from build123d import *

# Parameters (mm, degrees)
SKETCH1_W            = 20
SKETCH1_H            = 14.4
BOSS_EXTRUDE1_DEPTH  = 1.8
SKETCH2_W            = 20
SKETCH2_H            = 10
BOSS_EXTRUDE2_DEPTH  = 2.1
SKETCH3_W            = 30
SKETCH3_H            = 20
BOSS_EXTRUDE3_DEPTH  = 3
SKETCH4_W            = 2
SKETCH4_H            = 15
BOSS_EXTRUDE4_DEPTH  = 0.8
FILLET1_R            = 1.5
SKETCH5_W            = 27
SKETCH5_H            = 3
BOSS_EXTRUDE6_DEPTH  = 10
CUT_EXTRUDE1_DEPTH   = 40.819718733
SKETCH7_W            = 20
SKETCH7_H            = 4
BOSS_EXTRUDE7_DEPTH  = 4
SKETCH8_W            = 20
SKETCH8_H            = 4
BOSS_EXTRUDE8_DEPTH  = 4
FILLET3_R            = 2
FILLET2_R            = 1
FILLET4_R            = 1
SKETCH10_W           = 7
SKETCH10_H           = 4
BOSS_EXTRUDE10_DEPTH = 7
SKETCH11_W           = 3
SKETCH11_H           = 7
BOSS_EXTRUDE11_DEPTH = 3
FILLET5_R            = 2
FILLET6_R            = 1
FILLET7_R            = 3


# Some blends are built 0.0001 mm under size
with BuildPart() as part:
    # Sketch1 → Boss-Extrude1 (new body)
    with BuildSketch(Plane(origin=(0, 0, 0), x_dir=(1, 0, 0), z_dir=(0, 1, 0))):
        with Locations((10, -7.2)):
            Rectangle(SKETCH1_W, SKETCH1_H)
    extrude(amount=BOSS_EXTRUDE1_DEPTH)

    # Sketch2 → Boss-Extrude2 (add)
    with BuildSketch(Plane(origin=(0, 1.8, 0), x_dir=(1, 0, 0), z_dir=(0, 1, 0))):
        with Locations((10, -7.2)):
            Rectangle(SKETCH2_W, SKETCH2_H)
    extrude(amount=BOSS_EXTRUDE2_DEPTH)

    # Sketch3 → Boss-Extrude3 (add)
    with BuildSketch(Plane(origin=(0, 3.9, 0), x_dir=(1, 0, 0), z_dir=(0, 1, 0))):
        with Locations((15, -7.2)):
            Rectangle(SKETCH3_W, SKETCH3_H)
    extrude(amount=BOSS_EXTRUDE3_DEPTH)

    # Sketch4 → Boss-Extrude4 (add)
    with BuildSketch(Plane(origin=(0, 3.9, 0), x_dir=(-1, 0, 0), z_dir=(0, -1, 0))):
        with Locations((-28, -7.2)):
            Rectangle(SKETCH4_W, SKETCH4_H)
    extrude(amount=BOSS_EXTRUDE4_DEPTH)

    # Fillet1
    # the kernel refuses this fillet: 1.5 mm, written as the material it takes off along each edge
    with BuildSketch(Plane(origin=(27, 3.1, -3.61662479), x_dir=(0, 1, 0), z_dir=(0, 0, 1))) as fillet1_piece_1:
        with BuildLine():
            CenterArc((1.5, -1.326649916), FILLET1_R, 117.818139285, 62.181860715)
            Line((0, -1.326649916), (-0.03, -1.326649916))
            Line((-0.03, -1.326649916), (-0.03, 0))
            Line((-0.03, 0), (0, 0.03))
            ThreePointArc((0, 0.03), (0.4, 0.03), (0.786, 0.026532998))
            Line((0.786, 0.026532998), (0.8, 0))
        make_face()
    extrude(amount=21.633249581, mode=Mode.SUBTRACT)

    # Sketch5 → Boss-Extrude6 (add)
    with BuildSketch(Plane(origin=(0, 6.9, 0), x_dir=(1, 0, 0), z_dir=(0, 1, 0))):
        with Locations((13.5, 1.3)):
            Rectangle(SKETCH5_W, SKETCH5_H)
        with Locations((13.5, -15.7)):
            Rectangle(SKETCH5_W, SKETCH5_H)
    extrude(amount=BOSS_EXTRUDE6_DEPTH)

    # Sketch6 → Cut-Extrude1 (cut, through all)
    with BuildSketch(Plane.XY.offset(17.2)):
        with BuildLine():
            Line((1.325139576, 16.9), (25.674860424, 16.9))
            ThreePointArc((25.674860424, 16.9), (13.5, 10.331979326), (1.325139576, 16.9))
        make_face()
    extrude(amount=-CUT_EXTRUDE1_DEPTH, mode=Mode.SUBTRACT)

    # Sketch7 → Boss-Extrude7 (add)
    with BuildSketch(Plane(origin=(27, 0, 0), x_dir=(0, 0, -1), z_dir=(1, 0, 0))):
        with Locations((-7.2, 14.9)):
            Rectangle(SKETCH7_W, SKETCH7_H)
    extrude(amount=BOSS_EXTRUDE7_DEPTH)

    # Sketch8 → Boss-Extrude8 (add)
    with BuildSketch(Plane.ZY):
        with Locations((7.2, 14.9)):
            Rectangle(SKETCH8_W, SKETCH8_H)
    extrude(amount=BOSS_EXTRUDE8_DEPTH)

    # Fillet3
    fillet3_edges = [part.edges().sort_by_distance(p)[0] for p in [
        (27, 12.9, 15.7),
        (27, 12.9, -1.3),
        (0, 12.9, 15.7),
        (0, 12.9, -1.3),
    ]]
    fillet(fillet3_edges, radius=FILLET3_R)

    # Fillet2
    fillet2_edges = [part.edges().sort_by_distance(p)[0] for p in [
        (-3, 12.9, -2.8),
        (-3, 12.9, 17.2),
        (0, 7.4, -2.8),
        (0, 7.4, 17.2),
        (-0.585786438, 12.314213562, 17.2),
        (-0.585786438, 12.314213562, -2.8),
        (30, 5.4, 17.2),
        (30, 5.4, -2.8),
        (0, 0.9, 0),
        (20, 0.9, 0),
        (20, 0.9, 14.4),
        (0, 0.9, 14.4),
    ]]
    fillet(fillet2_edges, radius=FILLET2_R)

    # Fillet4
    fillet4_edges = [part.edges().sort_by_distance(p)[0] for p in [
        (30, 12.9, 17.2),
        (30, 12.9, -2.8),
        (27, 8.9, -2.8),
        (27, 8.9, 17.2),
        (27.585786438, 12.314213562, -2.8),
        (27.585786438, 12.314213562, 17.2),
    ]]
    fillet(fillet4_edges, radius=FILLET4_R)

    # Sketch10 → Boss-Extrude10 (add)
    with BuildSketch(Plane.ZY.offset(4)):
        with Locations((7.2, 14.9)):
            Rectangle(SKETCH10_W, SKETCH10_H)
    extrude(amount=BOSS_EXTRUDE10_DEPTH)

    # Sketch11 → Boss-Extrude11 (add)
    with BuildSketch(Plane(origin=(0, 12.9, 0), x_dir=(-1, 0, 0), z_dir=(0, -1, 0))):
        with Locations((9.5, -7.2)):
            Rectangle(SKETCH11_W, SKETCH11_H)
    extrude(amount=BOSS_EXTRUDE11_DEPTH)

    # Fillet5
    fillet5_edges = [part.edges().sort_by_distance(p)[0] for p in [
        (-8, 12.9, 7.2),
    ]]
    fillet(fillet5_edges, radius=FILLET5_R)

    # Fillet6
    fillet6_edges = [part.edges().sort_by_distance(p)[0] for p in [
        (-11, 9.9, 7.2),
        (-8, 9.9, 7.2),
    ]]
    fillet(fillet6_edges, radius=FILLET6_R - 0.0001)  # a hair under: the kernel refuses the full size

    # Fillet7
    fillet7_edges = [part.edges().sort_by_distance(p)[0] for p in [
        (-11, 16.9, 7.2),
    ]]
    fillet(fillet7_edges, radius=FILLET7_R)


solid = part.part
The listing builds one solid part. Answer for the finished solid, in the listing's coordinates (mm). A direction names the side the tool comes from. Give positions to 0.01 mm unless a question says otherwise; leave off trailing zeros. Write each loop counter-clockwise with the first axis right and the second up, starting at its lowest first coordinate (ties: lowest second). Pieces come first, ordered by that corner, then holes.
Item 1: Find the intervals of material crossed by line 1 along X through (y, z) = (13.25, 13.25); line 2 along Z through (x, y) = (16.5, 10.25); line 3 along Y through (x, z) = (5.5, 13), in increasing order.
Item 2: Section B-B, the plane z = 7.25 is taken. Count the separate pieces of the cut face and the enclosed holes in it, plus the area to 3 significant figures.
Item 3: Section D-D, the plane x = 8.5 is taken. Write down the section's boundary in (y, z), plus the area to 3 significant figures.
Item 4: Section C-C, the plane y = 6 is taken. Write down the section's boundary in (x, z).
Item 5: Determine the mould class of faces 5 (the flat face through (15, 6.9, 7)), 6 (the flat face through (14, 9, -2.8)), 7 (the flat face through (29, 16.9, 7)) for opening direction Y: released by +Y, released by -Y, zero draft, split by the parting line, or undercut.
Item 6: Flat-ended cylindrical pins translate along their axes: P1, Ø5.5, axis at y = 6.5, z = 6.5, coming from the -X side; P2, Ø3, axis at x = 29, z = 4, coming from the -Y side; P3, Ø5.5, axis at x = -7.5, y = 12, coming from the -Z side. Find the tip coordinate at first contact, or state that the pin passes through.
Item 7: Which of the six approach directions +Z, -Z, +X, -X, +Y, -Y give full straight-line access (tool end or side, diameter ignored) to faces 1 (the flat face through (-4, 15, 14)), 2 (the cylindrical face through (26.715, 8.928, 16.899)), 3 (the flat face through (10, 1, 0)), 4 (the cylindrical face through (27.57, 12.3, -0.81))?
Item 8: Section A-A, the plane y = 8.5 is taken. Write down the section's boundary in (x, z), plus the area to 3 significant figures.
Completed:
1. line 1: x = -4 to 0, 27 to 31
1. line 2: z = -2.8 to 0.2, 14.2 to 17.2
1. line 3: y = 0 to 1.8, 3.9 to 6.9
2. separate pieces: 3
2. enclosed holes: 0
2. area: 237 mm2
3. outline: (0, 0) - (1.8, 0) - (1.8, 2.2) - (3.9, 2.2) - (3.9, -2.8) - (11.22, -2.8) - (11.22, 0.2) - (6.9, 0.2) - (6.9, 14.2) - (11.22, 14.2) - (11.22, 17.2) - (3.9, 17.2) - (3.9, 12.2) - (1.8, 12.2) - (1.8, 14.4) - (0, 14.4) - close
3. area: 133 mm2
4. outline: (0, -1.8) arc R1 ccw to (1, -2.8) - (29, -2.8) arc R1 ccw to (30, -1.8) - (30, 16.2) arc R1 ccw to (29, 17.2) - (1, 17.2) arc R1 ccw to (0, 16.2) - close
5. face 5: undercut
5. face 6: zero draft
5. face 7: released by +Y
6. P1: stops at x = 0
6. P2: stops at y = 3.1
6. P3: stops at z = 3.7
7. face 1: +Z, -X, +Y, -Y
7. face 2: +Z, +X
7. face 3: -Z, +X, -X, -Y
7. face 4: +Z, -Z, +X
8. outline: (0, -1.8) arc R1 ccw to (1, -2.8) - (26, -2.8) arc R1 ccw to (27, -1.8) - (27, 0.2) - (0, 0.2) - close; (0, 14.2) - (27, 14.2) - (27, 16.2) arc R1 ccw to (26, 17.2) - (1, 17.2) arc R1 ccw to (0, 16.2) - close
8. area: 161 mm2
